```python
from build123d import *

# Parameters (mm, degrees)
F0_R     = 1.6
F1_DEPTH = 4
F2_R     = 16
F2_R_2   = 7.5
F2_W     = 25
F2_H     = 4
F3_DEPTH = 3


with BuildPart() as f1:
    # F0 (on Top) → F1 (new body)
    with BuildSketch(Plane.XY):
        with BuildLine():
            ThreePointArc((0, 1.6), (1.1313708499, 1.1313708499), (1.6, 0))
            ThreePointArc((1.6, 0), (1.1313708499, -1.1313708499), (0, -1.6))
            Line((0, -1.6), (0, -27))
            Line((0, -27), (-13.0766968306, -27))
            ThreePointArc((-13.0766968306, -27), (15.9326566379, -25.4194896184), (30, 0))
            ThreePointArc((30, 0), (15.9326566379, 25.4194896184), (-13.0766968306, 27))
            Line((-13.0766968306, 27), (0, 27))
            Line((0, 27), (0, 26.6))
            ThreePointArc((0, 26.6), (1.1313708499, 26.1313708499), (1.6, 25))
            ThreePointArc((1.6, 25), (1.1313708499, 23.8686291501), (0, 23.4))
            Line((0, 23.4), (0, 1.6))
        make_face()
        with Locations((25, 0)):
            Circle(F0_R, mode=Mode.SUBTRACT)
        with BuildLine():
            ThreePointArc((0, -1.6), (-1.6, 0), (0, 1.6))
            Line((0, 1.6), (0, 23.4))
            ThreePointArc((0, 23.4), (-1.6, 25), (0, 26.6))
            Line((0, 26.6), (0, 27))
            Line((0, 27), (-13.0766968306, 27))
            ThreePointArc((-13.0766968306, 27), (-25.4194896184, 15.9326566379), (-30, 0))
            ThreePointArc((-30, 0), (-25.4194896184, -15.9326566379), (-13.0766968306, -27))
            Line((-13.0766968306, -27), (0, -27))
            Line((0, -27), (0, -1.6))
        make_face()
        with Locations((-25, 0)):
            Circle(F0_R, mode=Mode.SUBTRACT)
        with BuildLine():
            Line((-40, -27), (-13.0766968306, -27))
            ThreePointArc((-13.0766968306, -27), (-25.4194896184, -15.9326566379), (-30, 0))
            ThreePointArc((-30, 0), (-32, -2), (-34, 0))
            Line((-34, 0), (-40, 0))
            Line((-40, 0), (-40, -27))
        make_face()
        with BuildLine():
            ThreePointArc((-34, 0), (-32, 2), (-30, 0))
            ThreePointArc((-30, 0), (-25.4194896184, 15.9326566379), (-13.0766968306, 27))
            Line((-13.0766968306, 27), (-40, 27))
            Line((-40, 27), (-40, 0))
            Line((-40, 0), (-34, 0))
        make_face()
    extrude(amount=-F1_DEPTH)

    # F2 (on Top) → F3 (join)
    with BuildSketch(Plane.XY):
        Circle(F2_R)
        Circle(F2_R_2, mode=Mode.SUBTRACT)
        with Locations((-27.5, -25)):
            Rectangle(F2_W, F2_H)
        with Locations((-27.5, 25)):
            Rectangle(F2_W, F2_H)
    extrude(amount=F3_DEPTH)


solid = f1.part
```
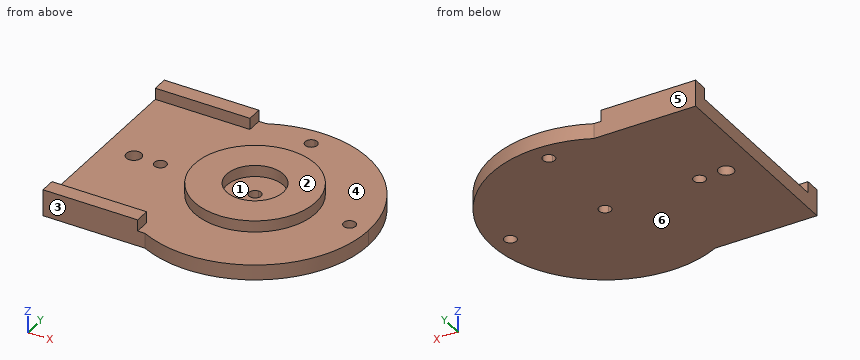
Source: CAD feature listing. Evaluate the final solid. Frame: model axes, mm. Face numbers are marked on the shaded views. A direction names the side the tool comes from. Round coordinates to 2 decimals unless told otherwise and drop trailing zeros. Order: outer loops, then holes, each group sorted by start corner. A loop starts at its lowest first (then second) coordinate and runs counter-clockwise, first axis right, second up. Notation, with made-up numbers: (1.25, 16.25) -> (10.25, 16.25) arc R25 cw to (10.25, 34.25) -> close; hole circle Ø3 at (74.5, -17). An arc over 180 degrees is marked (long way). One line per item, written item: value. Start each with the question number.
Q1. Section query B-B (x = -32). Return the cut outline in (y, z), plus the area to 3 significant figures.
Q2. Section query A-A (z = 1). Return the cut outline in (x, y), plus the area to 3 significant figures.
Q3. Draft query along Y for the marked faces 4, 5 and 6. Return one class per face: pulls with the +Y half, pulls with the -Y half, needs draft (parallel to the pull), parting line crosses it, or undercut.
Q4. Section query D-D (x = -25). Return the cut outline in (y, z).
Q5. Material intervals for probe 1 along Y at (x, z) = (0, 1.2); probe 2 along Y at (x, z) = (-32, -2.4); probe 3 along Y at (x, z) = (-1, -2.75), sorted ascending.
Q6. Section query C-C (z = -2.25). Return the cut outline in (x, y).
Q7. Pin query (flat end, axial travel): pin 1 (2 mm diameter, centred on y = 5, z = -1.5, fed in from +X); pin 2 (2.5 mm diameter, centred on x = -28, z = 1.5, fed in from -Y); pin 3 (4.5 mm diameter, centred on x = -3, y = 1.5, fed in from +Z). Return the tip coordinate at first contact, or that it passes through.
Q8. Access query for the marked faces 1, 2 and 3. Directions: +Z, -Z, +X, -X, +Y, -Y. A direction counts if a zero-diameter tool reaches every point of the face in a straight line with its end or side. Return the directions, or none.
Findings below:
1. outline: (-27, -4) -> (-2, -4) -> (-2, 0) -> (-23, 0) -> (-23, 3) -> (-27, 3) -> close; (2, -4) -> (27, -4) -> (27, 3) -> (23, 3) -> (23, 0) -> (2, 0) -> close
1. area: 224 mm²
2. outline: (-40, -27) -> (-15, -27) -> (-15, -23) -> (-40, -23) -> close; (-40, 23) -> (-15, 23) -> (-15, 27) -> (-40, 27) -> close; circle Ø32 at (0, 0); hole circle Ø15 at (0, 0)
2. area: 828 mm²
3. face 4: undercut
3. face 5: pulls with the +Y half
3. face 6: needs draft
4. outline: (-27, -4) -> (-1.6, -4) -> (-1.6, 0) -> (-23, 0) -> (-23, 3) -> (-27, 3) -> close; (1.6, -4) -> (27, -4) -> (27, 3) -> (23, 3) -> (23, 0) -> (1.6, 0) -> close
5. probe 1: -16 to -7.5, 7.5 to 16
5. probe 2: -27 to -2, 2 to 27
5. probe 3: -29.98 to -1.25, 1.25 to 23.75, 26.25 to 29.98
6. outline: (-40, -27) -> (-13.08, -27) arc R30 ccw (long way) to (-13.08, 27) -> (-40, 27) -> close; hole circle Ø4 at (-32, 0); hole circle Ø3.2 at (-25, 0); hole circle Ø3.2 at (0, 0); hole circle Ø3.2 at (0, 25); hole circle Ø3.2 at (25, 0)
7. pin 1: x = 29.73
7. pin 2: y = -27
7. pin 3: z = 0
8. face 1: +Z
8. face 2: +Z, +X, -X, +Y, -Y
8. face 3: +Z, -Z, -X, -Y
